Verification items for this drawing (mm, ordinates from the low corner). Give positions to 0.01 mm unless a question says otherwise; leave off trailing zeros. Loops run counter-clockwise (first coordinate to the right, second up) from the corner with the lowest first, then second, coordinate; pieces in that order, holes last. Notation, with made-up numbers: M 56,46 L 65,46 A16 ccw 65,75 Z; hole C 36.5,74.5 d6. An arc over 180 degrees is marked long. Use one line per item in the form item = value.
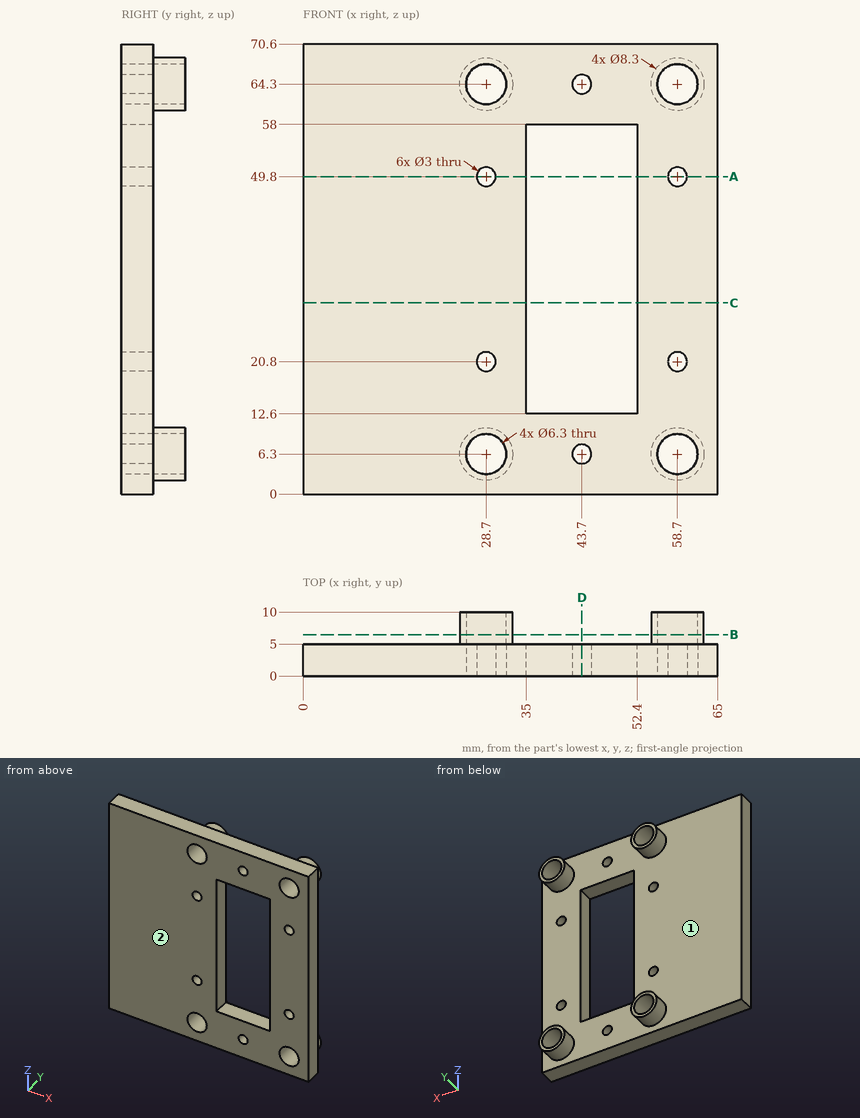
1) Section check D-D (x = 43.7). Record the cut outline in (y, z), then the cut area to 3 significant figures.
Evaluation:
outline = M 0,0 L 5,0 L 5,4.8 L 0,4.8 Z; M 0,7.8 L 5,7.8 L 5,12.6 L 0,12.6 Z; M 0,58 L 5,58 L 5,62.8 L 0,62.8 Z; M 0,65.8 L 5,65.8 L 5,70.6 L 0,70.6 Z
area = 96.0 mm^2
2) Section check C-C (z = 30). Record the cut outline in (x, y), then the cut area to 3 significant figures.
Evaluation:
outline = M 0,0 L 35,0 L 35,5 L 0,5 Z; M 52.4,0 L 65,0 L 65,5 L 52.4,5 Z
area = 238 mm^2
3) Scan lines: line 1 (Z direction, x = 58.7, y = 1.6); line 2 (X direction, y = 6.25, z = 64.3); line 3 (X direction, y = 3.8, z = 64.3). Record each from-to range of solid material in increasing order.
Evaluation:
line_1 = 0 to 3.15, 9.45 to 19.3, 22.3 to 48.3, 51.3 to 61.15, 67.45 to 70.6
line_2 = 24.55 to 25.55, 31.85 to 32.85, 54.55 to 55.55, 61.85 to 62.85
line_3 = 0 to 25.55, 31.85 to 42.2, 45.2 to 55.55, 61.85 to 65
4) Release check for a two-part mould opening along Z. For the marked faces 1 and 2 record: pulls with the +Z half, pulls with the -Z half, needs draft (parallel to the pull), parting line crosses it, or undercut.
Evaluation:
face_1 = undercut
face_2 = needs draft
5) Section check A-A (z = 49.8). Record the cut outline in (x, y), then the cut area to 3 significant figures.
Evaluation:
outline = M 0,0 L 27.2,0 L 27.2,5 L 0,5 Z; M 30.2,0 L 35,0 L 35,5 L 30.2,5 Z; M 52.4,0 L 57.2,0 L 57.2,5 L 52.4,5 Z; M 60.2,0 L 65,0 L 65,5 L 60.2,5 Z
area = 208 mm^2
6) Depth check by flat-ended pin: pin 1 Ø1 at (x, z) = (23.5, 52) entering from +Y. Enter the tip coordinate at first touch or a pass-through.
Evaluation:
pin_1 = 5
7) Section check B-B (y = 6.5). Record the cut outline in (x, z), then the cut area to 3 significant figures.
Evaluation:
outline = C 28.7,6.3 d8.3; C 28.7,64.3 d8.3; C 58.7,6.3 d8.3; C 58.7,64.3 d8.3; hole C 28.7,6.3 d6.3; hole C 28.7,64.3 d6.3; hole C 58.7,6.3 d6.3; hole C 58.7,64.3 d6.3
area = 91.7 mm^2
